Check sheet for the drawn part. Datum: minimum x, y, z corner. Units: mm. A direction names the side the tool comes from. Coordinates: 2 decimals unless noted, no trailing zeros. Write each loop counter-clockwise with the first axis right and the second up, starting at its lowest first coordinate (ties: lowest second). Pieces come first, ordered by that corner, then holes. Notation, with made-up numbers: (-6, 65) -> (7, 65) arc R8 cw to (7, 70) -> close; hole circle Ø10 at (-9, 56). An arc over 180 degrees is marked (long way). Answer in a Markdown table with one row per item.
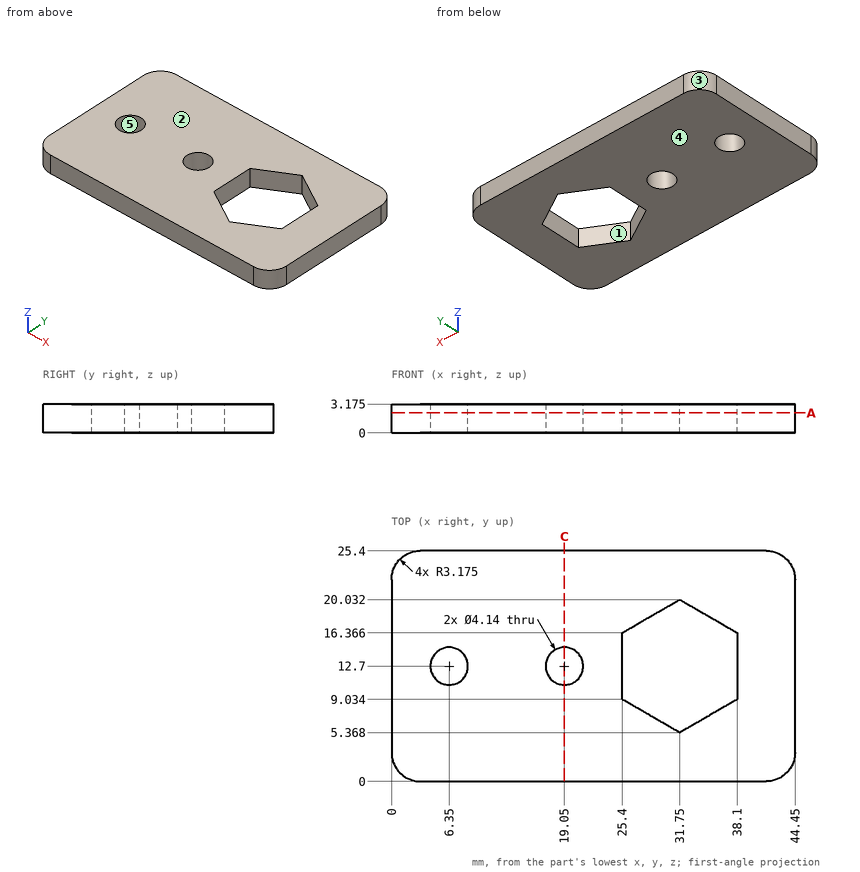
1. Sectioned sample at A-A, the plane z = 2.2. Count the separate pieces of the cut face and the enclosed holes in it, and give its area (3 significant figures).
Findings below:
| item | result |
|---|---|
| separate pieces | 1 |
| enclosed holes | 3 |
| area | 954 mm² |
2. Go/stop test with a flat-tipped pin: pin 1 (2.5 mm diameter, centred on x = 6.35, y = 12.7, fed in from -Z). Record where the tip stops, or that it passes through.
Findings below:
| item | result |
|---|---|
| pin 1 | passes through |
3. Sectioned sample at C-C, the plane x = 19.05. Record the cut outline in (y, z) (1 decimal), and give its area (3 significant figures).
Findings below:
| item | result |
|---|---|
| outline | (0, 0) -> (10.6, 0) -> (10.6, 3.2) -> (0, 3.2) -> close; (14.8, 0) -> (25.4, 0) -> (25.4, 3.2) -> (14.8, 3.2) -> close |
| area | 67.5 mm² |
4. Material ranges on probe 1 along Y at (x, z) = (19.05, 2.35); probe 2 along X at (y, z) = (10.25, 1.2); probe 3 along X at (y, z) = (6.25, 1.4), recorded low to high. Write a range as from..to.
Findings below:
| item | result |
|---|---|
| probe 1 | y = 0..10.63, 14.77..25.4 |
| probe 2 | x = 0..25.4, 38.1..44.45 |
| probe 3 | x = 0..30.22, 33.28..44.45 |
5. Access from +Z, -Z, +X, -X, +Y, -Y to the whole of each face (thin tool, end or side, straight path). Record for the marked faces 1 and 2.
Findings below:
| item | result |
|---|---|
| face 1 | +Z, -Z |
| face 2 | +Z, +X, -X, +Y, -Y |
6. Release check for a two-part mould opening along X. For the marked faces 3, 4 and 5 record: released by +X, released by -X, zero draft, split by the parting line, or undercut.
Findings below:
| item | result |
|---|---|
| face 3 | released by -X |
| face 4 | zero draft |
| face 5 | undercut |
